CAD build for the part. Positions are in the model's coordinates, mm. Face numbers are marked on the shaded views. Give positions to 0.01 mm unless a question says otherwise; leave off trailing zeros. Order: outer loops, then holes, each group sorted by start corner. A loop starts at its lowest first (then second) coordinate and runs counter-clockwise, first axis right, second up. Notation, with made-up numbers: M -19.75,29.25 L -15.75,29.25 A13 ccw -15.75,54.25 Z; hole C 5,-38.5 d3. An arc over 180 degrees is marked long. Put each result on its own line as item: value. Start each with the question number.
1) Cut at C-C (y = 1.3). Write the cut outline in (x, z), and give its area (3 significant figures).
2) Pin check, flat tips, straight feed: pin 1 (1 mm diameter, centred on x = -6, y = 2.5, fed in from +Z); pin 2 (1 mm diameter, centred on x = 1, y = 3, fed in from +Z); pin 3 (2 mm diameter, centred on x = 6, z = 5, fed in from +Y). Stop position of each tip, or through.
3) Drill centre lines: line 1 (X direction, y = 0.35, z = -5.75); line 2 (X direction, y = 3.9, z = -1.25); line 3 (Z direction, x = -4.75, y = 0.75). Where is each one in solid material? Low to high. Write a range as [from, to].
4) Cut at B-B (z = 0). Write the cut outline in (x, y).
5) Two-plate mould, pull along X, no slides. Class the marked faces 1, 2 and 3: released by +X, released by -X, zero draft, split by the parting line, or undercut.
6) Cut at D-D (y = 2.3). Write the cut outline in (x, z).
7) Cut at A-A (x = 0). Write the cut outline in (y, z).
```python
from build123d import *

# Parameters (mm, degrees)
REDONDEO1_R = 2.5


with BuildPart() as part:
    # Croquis1 → Revolución1 (revolve)
    with BuildSketch(Plane.XY, mode=Mode.PRIVATE) as revoluci_n1_sk:
        Polygon((-7, 0.014889516), (-5.98143128, 4.539027855), (-6.528856455, 4.539027855), (-7.548007417, 3.479790211), (-9, 3.479790211), (-9, 0.014889516), align=None)
    revolve(revoluci_n1_sk.sketch.rotate(Axis((0, 13.059059278, 0), (0, -1, 0)), 270), axis=Axis((0, 13.059059278, 0), (0, -1, 0)))

    # Redondeo1
    redondeo1_edges = [part.edges().sort_by_distance(p)[0] for p in [
        (0, 3.479790211, -7.548007417),
    ]]
    fillet(redondeo1_edges, radius=REDONDEO1_R)


solid = part.part
```
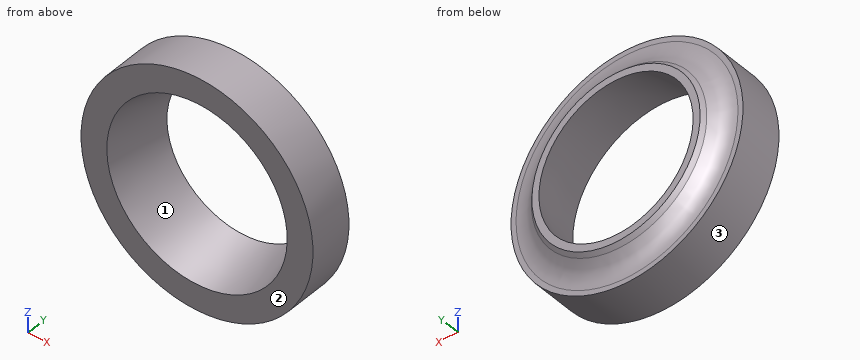
Solution:
1. outline: C 0,0 d18; hole C 0,0 d13.42
1. area: 113 mm²
2. pin 1: z = 7.12
2. pin 2: z = 8.99
2. pin 3: y = 4.25
3. line 1: [-6.92, -3.86], [3.86, 6.92]
3. line 2: [-7.12, -6], [6, 7.12]
3. line 3: [-7.64, -4.91], [4.91, 7.64]
4. outline: M -9,0.01 L -7,0.01 L -5.98,4.54 L -6.53,4.54 L -6.81,4.25 A2.5 cw -8.61,3.48 L -9,3.48 Z; M 5.98,4.54 L 7,0.01 L 9,0.01 L 9,3.48 L 8.61,3.48 A2.5 cw 6.81,4.25 L 6.53,4.54 Z
5. face 1: undercut
5. face 2: zero draft
5. face 3: split by the parting line
6. outline: C 0,0 d18; hole C 0,0 d12.97
7. outline: M 0.01,-9 L 3.48,-9 L 3.48,-8.61 A2.5 cw 4.25,-6.81 L 4.54,-6.53 L 4.54,-5.98 L 0.01,-7 Z; M 0.01,7 L 4.54,5.98 L 4.54,6.53 L 4.25,6.81 A2.5 cw 3.48,8.61 L 3.48,9 L 0.01,9 Z
